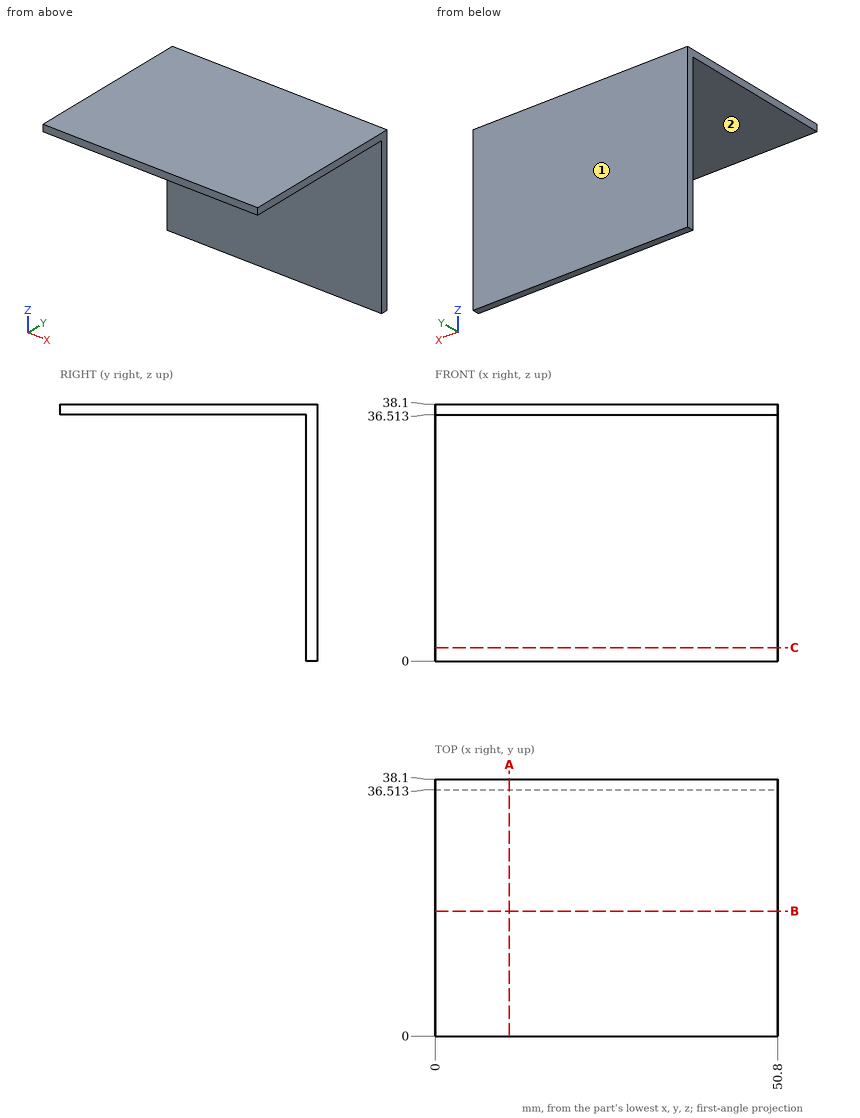
Part print with two shaded views. Sizes in mm from the minimum x, y, z corner. A direction names the side the tool comes from. Give positions to 0.01 mm unless a question says otherwise; leave off trailing zeros. Order: outer loops, then holes, each group sorted by start corner. A loop starts at its lowest first (then second) coordinate and runs counter-clockwise, first axis right, second up. Notation, with made-up numbers: M 23,-8.75 L 74,-8.75 A14 cw 74,3.25 Z; hole C -21.75,-11.5 d4. An arc over 180 degrees is marked long. Write item = value, one per line.
Q1. Flat gauge pins, fed straight in: pin 1 (11 mm diameter, centred on x = 16, y = 25.5, fed in from -Z); pin 2 (11 mm diameter, centred on x = 30, z = 21, fed in from -Y). Where does each tip first touch, or does it go through?
Derived:
pin_1 = 36.51
pin_2 = 36.51
Q2. Cut at B-B, the plane y = 18.5. List the corners of the cut face in (x, z).
Derived:
outline = M 0,36.51 L 50.8,36.51 L 50.8,38.1 L 0,38.1 Z
Q3. Drill centre line: line 1 (Y direction, x = 47.5, z = 3.5). Where is it in solid material? Low to high. Write a range as [from, to].
Derived:
line_1 = [36.51, 38.1]
Q4. Tool access for the marked faces 1 and 2: list every direction of +Z, -Z, +X, -X, +Y, -Y with a clear straight run to the whole face (end or side of a thin tool).
Derived:
face_1 = +Z, -Z, +X, -X, +Y
face_2 = -Z, +X, -X, -Y
Q5. Cut at A-A, the plane x = 11. List the corners of the cut face in (y, z).
Derived:
outline = M 0,36.51 L 36.51,36.51 L 36.51,0 L 38.1,0 L 38.1,38.1 L 0,38.1 Z
